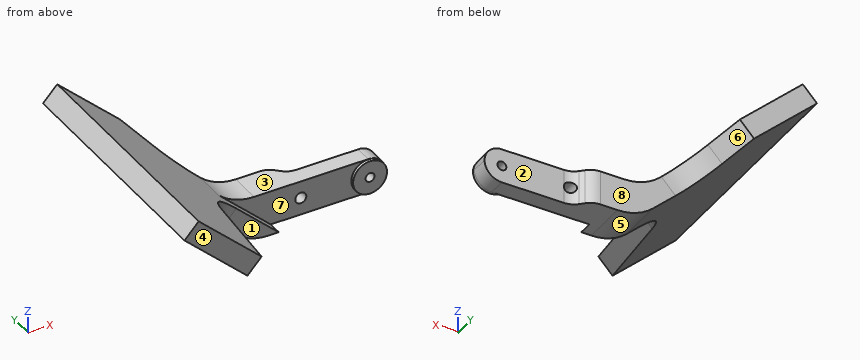
```python
from build123d import *

# Parameters (mm, degrees)
BOSS_EXTRUDE1_DEPTH = 5
FILLET1_R           = 5
SKETCH2_R           = 1.2999999999999945
CUT_EXTRUDE1_DEPTH  = 10
BOSS_EXTRUDE2_DEPTH = 20
BOSS_EXTRUDE3_DEPTH = 45
BOSS_EXTRUDE4_DEPTH = 6
SKETCH6_R           = 4.900000000000002
SKETCH6_R_2         = 1.299999999999994
BOSS_EXTRUDE5_DEPTH = 0.9
BOSS_EXTRUDE6_DEPTH = 3.9999999999999964
BOSS_EXTRUDE7_DEPTH = 3.9999999999999964
FILLET2_R           = 15
FILLET7_SIZE        = 5
FILLET8_R           = 5
SKETCH11_R          = 1.6000000000000019
CUT_EXTRUDE2_DEPTH  = 10


# Some blends are built 0.0001 mm under size
with BuildPart() as part:
    # Sketch1 → Boss-Extrude1 (new body)
    with BuildSketch(Plane(origin=(0, 0, 0), x_dir=(1, 0, 0), z_dir=(0, 1, 0))):
        Polygon((4.091990160374978, 5.611877790284978), (0, 10), (0, 1.79603523340848), align=None)
        Polygon((0, 1.79603523340848), (0, 10), (-42.4185146939121, -29.55590488362469), (-38.32652453353713, -33.94402709333974), (-1.9260119864091507, 0), align=None)
        Polygon((42, 10), (0, 10), (4.091990160374978, 5.611877790284978), (0, 1.7960352334084817), (0, 0), (42, 0), align=None)
        Polygon((0, 0), (0, 1.79603523340848), (-1.9260119864091507, 0), align=None)
    extrude(amount=BOSS_EXTRUDE1_DEPTH)

    # Fillet1
    fillet1_edges = [part.edges().sort_by_distance(p)[0] for p in [
        (42, 2.5, 0),
        (42, 2.5, -10),
    ]]
    fillet(fillet1_edges, radius=FILLET1_R - 0.0001)  # a hair under: the kernel refuses the full size

    # Sketch2 → Cut-Extrude1 (cut)
    with BuildSketch(Plane(origin=(0, 5, 0), x_dir=(1, 0, 0), z_dir=(0, 1, 0))):
        with Locations(Location((37.00000000000001, 4.999999999999989, 0), (0, 0, 270))):
            Circle(SKETCH2_R)
    extrude(amount=-CUT_EXTRUDE1_DEPTH, mode=Mode.SUBTRACT)

    # Sketch3 → Boss-Extrude2 (add)
    with BuildSketch(Plane(origin=(0, 5, 0), x_dir=(1, 0, 0), z_dir=(0, 1, 0))):
        Polygon((-42.4185146939121, -29.55590488362471), (-38.32652453353713, -33.94402709333974), (-20.126268259973138, -16.97201354666987), (-24.21825842034811, -12.583891336954824), align=None)
    extrude(amount=BOSS_EXTRUDE2_DEPTH)

    # Sketch4 → Boss-Extrude3 (add)
    with BuildSketch(Plane.XZ):
        Polygon((-42.4185146939121, 29.55590488362471), (-38.32652453353713, 33.94402709333974), (-20.126268259973134, 16.972013546669885), (-24.218258420348107, 12.583891336954828), align=None)
    extrude(amount=BOSS_EXTRUDE3_DEPTH)

    # Sketch5 → Boss-Extrude4 (add)
    with BuildSketch(Plane(origin=(-4.987820251299118, 0, -5.348782368720677), x_dir=(-0.7313537016191739, 0, 0.6819983600624947), z_dir=(-0.6819983600624948, 0, -0.731353701619174))):
        Polygon((26.29430619749914, -45), (26.29430619749914, 0), (13.888976828400956, 0), align=None)
        Polygon((13.888976828400958, 5), (26.29430619749914, 25), (26.29430619749914, 5), align=None)
    extrude(amount=-BOSS_EXTRUDE4_DEPTH)

    # Sketch6 → Boss-Extrude5 (add)
    with BuildSketch(Plane.XZ):
        with Locations(Location((37.00000000000001, -4.999999999999989, 0), (0, 0, 90))):
            Circle(SKETCH6_R)
        with Locations(Location((37.00000000000001, -4.999999999999989, 0), (0, 0, 90))):
            Circle(SKETCH6_R_2, mode=Mode.SUBTRACT)
    extrude(amount=BOSS_EXTRUDE5_DEPTH)

    # Sketch8 → Boss-Extrude6 (add)
    with BuildSketch(Plane.XZ):
        Polygon((0, -10), (-19.681916643400598, 8.353684194074795), (-15.589926483025625, 12.741806403789838), (8.797675113837775, -10), align=None)
    extrude(amount=BOSS_EXTRUDE6_DEPTH)

    # Sketch9 → Boss-Extrude7 (add)
    with BuildSketch(Plane(origin=(0, 5, 0), x_dir=(1, 0, 0), z_dir=(0, 1, 0))):
        Polygon((0, 10), (-20.085147023573704, -8.729702606775238), (-16.79961762354496, -13.869861641891177), (-1.92601198640914, -7.11e-15), (17.950520425486616, 5.22e-15), (17.950520425486616, 10), align=None)
    extrude(amount=BOSS_EXTRUDE7_DEPTH)

    # Fillet2
    fillet2_edges = [part.edges().sort_by_distance(p)[0] for p in [
        (-14.914116497044613, 8.999999999999996, 8.009621013204297),
        (-1.9260119864091478, 4.499999999999998, 2.06e-15),
        (0, 2.5, -10),
        (-13.906040546611829, -3.9999999999999973, 7.069574981453184),
    ]]
    fillet(fillet2_edges, radius=FILLET2_R)

    # Fillet7
    # the kernel refuses this chamfer: 5 mm, written as the material it takes off along each edge
    with BuildSketch(Plane(origin=(17.950520425486616, 8.999999999999996, 12.858414939829549), x_dir=(0.027495876610586317, -0.9996219169112968, 0), z_dir=(0, 0, -1))) as fillet7_piece_1_section:
        Polygon((FILLET7_SIZE * 0.999621916911, FILLET7_SIZE * 0.0274958766106), (-FILLET7_SIZE * 0.0274958766106, FILLET7_SIZE * 0.999621916911), (0, 0), align=None)
    fillet7_piece_1 = extrude(amount=35.71682987965911, mode=Mode.PRIVATE)
    fillet7_piece_1 = split(fillet7_piece_1, bisect_by=Plane(origin=(16.221928363932022, 5, -5.000000000000004), z_dir=(0, 1, 0)), keep=Keep.TOP, mode=Mode.PRIVATE)
    add(fillet7_piece_1, mode=Mode.SUBTRACT)

    # Fillet8
    fillet8_edges = [part.edges().sort_by_distance(p)[0] for p in [
        (12.95052042548848, 8.999999999998002, -5.000000000000002),
        (16.950520425489678, 5, -4.999999999999999),
    ]]
    fillet(fillet8_edges, radius=FILLET8_R)

    # Sketch11 → Cut-Extrude2 (cut)
    with BuildSketch(Plane(origin=(0, 0, 0), x_dir=(-1, 0, 0), z_dir=(0, -1, 0))):
        with Locations(Location((-17.499999999999993, 5.000000000000053, 0), (0, 0, 90))):
            Circle(SKETCH11_R)
    extrude(amount=-CUT_EXTRUDE2_DEPTH, mode=Mode.SUBTRACT)


solid = part.part
```
The listing builds one solid part. Answer for the finished solid, in the listing's coordinates (mm). Face numbers are marked on the shaded views. A direction names the side the tool comes from. Round coordinates to 2 decimals unless told otherwise and drop trailing zeros. Order: outer loops, then holes, each group sorted by start corner. A loop starts at its lowest first (then second) coordinate and runs counter-clockwise, first axis right, second up. Notation, with made-up numbers: (-5.75, -12.75) - (3.25, -12.75) arc R23 ccw to (3.25, 18.25) - close; hole circle Ø3 at (19, -28.75). An arc over 180 degrees is marked (long way). Put each result on its own line as item: value. Start each with the question number.
(1) Find section C-C (z = 28). Give the vertices of the cut face in (x, y).
(2) For the marked faces 1, 2, 3 and 4, determine the directions among +Z, -Z, +X, -X, +Y, -Y from which every point of the face is accessible in a straight line to the end or side of a thin tool.
(3) Given P1, Ø2.5, axis at x = 22.5, y = 3, coming from the +Z side; P2, Ø8, axis at x = 26, z = -5, coming from the +Y side; P3, Ø5, axis at y = -20.5, z = 12.5, coming from the +X side, each flat-ended and moving along its own axis, determine where each tip first touches the part or whether it passes through.
(4) Straight lines are drawn through the part: probe 1 along X at (y, z) = (4, -5); probe 2 along Y at (x, z) = (2, -5); probe 3 along Z at (x, y) = (17, 4). For each, find the intervals that lie inside material, in ascending order. Write a range as from..to.
(5) Determine the mould class of the marked faces 5, 6, 7 and 8 for opening direction X: released by +X, released by -X, zero draft, split by the parting line, or undercut.
(6) Find section B-B (y = 12.5). Give the vertices of the cut face in (x, z).
(7) Find section A-A (x = 17.5). Give the vertices of the cut face in (y, z), plus the area to 3 significant figures.
Reply:
1. outline: (-40.75, -45) - (-31.95, -45) - (-31.95, 25) - (-40.75, 25) - close
2. face 1: -Z, +X, -Y
2. face 2: +Z, -Z, +X, +Y
2. face 3: +Z, +X, +Y, -Y
2. face 4: +Z, -Z, +X, -X, -Y
3. P1: z = 0
3. P2: y = 5
3. P3: x = -14.7
4. probe 1: -5.36..15.9, 19.1..35.7, 38.3..42
4. probe 2: -4..9
4. probe 3: -10..-6.52, -3.48..0
5. face 5: released by -X
5. face 6: released by +X
5. face 7: undercut
5. face 8: zero draft
6. outline: (-42.42, 29.56) - (-17.9, 6.69) - (-13.81, 11.08) - (-38.33, 33.94) - close
7. outline: (0, -10) - (5.24, -10) - (5.24, -6.6) - (0, -6.6) - close; (0, -3.4) - (5.24, -3.4) - (5.24, 0) - (0, 0) - close
7. area: 35.6 mm^2
